Input: part model. Units: mm. Frame: model coordinates. Face numbers are marked on the shaded views. A direction names the side the tool comes from. Coordinates: 2 decimals unless noted, no trailing zeros. Order: outer loops, then holes, each group sorted by start corner. A loop starts at its lowest first (then second) coordinate and runs counter-clockwise, first axis right, second up. Notation, with made-up numbers: (68, 74.5) -> (98, 74.5) arc R26 cw to (98, 95.5) -> close; hole circle Ø7 at (-32, 37). An arc over 180 degrees is marked (long way). One line per question, with ' | ' between items.
```python
from build123d import *

# Parameters (mm, degrees)
SKETCH1_R           = 40
BOSS_EXTRUDE1_DEPTH = 3
SKETCH2_R           = 30
BOSS_EXTRUDE2_DEPTH = 18
SKETCH3_R           = 1.625
SKETCH3_R_2         = 11.5
SKETCH3_R_3         = 2.5
CUT_EXTRUDE1_DEPTH  = 61.340699366


with BuildPart() as part:
    # Sketch1 → Boss-Extrude1 (new body)
    with BuildSketch(Plane.XY):
        Circle(SKETCH1_R)
    extrude(amount=BOSS_EXTRUDE1_DEPTH)

    # Sketch2 → Boss-Extrude2 (add)
    with BuildSketch(Plane.XY.offset(3)):
        Circle(SKETCH2_R)
    extrude(amount=BOSS_EXTRUDE2_DEPTH)

    # Sketch3 → Cut-Extrude1 (cut, through all)
    with BuildSketch(Plane.XY.offset(21)):
        with Locations((0, 20)):
            Circle(SKETCH3_R)
        with Locations((17.320508076, -10)):
            Circle(SKETCH3_R)
        with Locations((-17.320508076, -10)):
            Circle(SKETCH3_R)
        Circle(SKETCH3_R_2)
        with Locations((0, -20)):
            Circle(SKETCH3_R_3)
    extrude(amount=-CUT_EXTRUDE1_DEPTH, mode=Mode.SUBTRACT)


solid = part.part
```
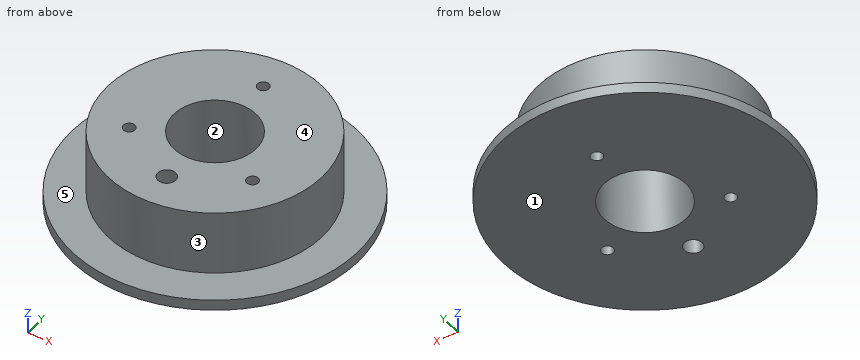
1. Pin query (flat end, axial travel): pin 1 Ø3 at (x, y) = (-17.32, -10) entering from +Z; pin 2 Ø4 at (y, z) = (6.5, 11.5) entering from -X; pin 3 Ø10 at (y, z) = (26.5, 9.5) entering from +X; pin 4 Ø4 at (x, z) = (-27, 15) entering from -Y. Return the tip coordinate at first contact, or that it passes through.
Recorded:
pin 1: passes through | pin 2: stops at x = -29.66 | pin 3: stops at x = 20.92 | pin 4: stops at y = -16.58
2. Mould query, pull axis X, two halves, no side actions, for the marked faces 1, 2 and 3. Classes: released by +X, released by -X, zero draft, split by the parting line, or undercut.
Recorded:
face 1: zero draft | face 2: undercut | face 3: split by the parting line
3. Access query for the marked faces 4 and 5. Directions: +Z, -Z, +X, -X, +Y, -Y. A direction counts if a zero-diameter tool reaches every point of the face in a straight line with its end or side. Return the directions, or none.
Recorded:
face 4: +Z, +X, -X, +Y, -Y | face 5: +Z
4. Cut plane A-A, the plane x = 0. Return loops of the section in (y, z) (3 decimals).
Recorded:
outline: (-40, 0) -> (-22.5, 0) -> (-22.5, 21) -> (-30, 21) -> (-30, 3) -> (-40, 3) -> close; (-17.5, 0) -> (-11.5, 0) -> (-11.5, 21) -> (-17.5, 21) -> close; (11.5, 0) -> (18.375, 0) -> (18.375, 21) -> (11.5, 21) -> close; (21.625, 0) -> (40, 0) -> (40, 3) -> (30, 3) -> (30, 21) -> (21.625, 21) -> close
5. Ray query, line 1 (Y direction, x = 0, z = 10) (3 decimals); line 2 (Y direction, x = -2, z = 6.25); line 3 (Y direction, x = -16, z = 15.5). Return the intervals inside material, ascending. Write a range as [from, to].
Recorded:
line 1: y = [-30, -22.5], [-17.5, -11.5], [11.5, 18.375], [21.625, 30] | line 2: y = [-29.93, -21.5], [-18.5, -11.32], [11.32, 29.93] | line 3: y = [-25.38, -10.95], [-9.05, 25.38]
6. Cut plane B-B, the plane z = 11.75. State how many separate pieces and enclosed holes the cut face has, and give its area (3 significant figures).
Recorded:
separate pieces: 1 | enclosed holes: 5 | area: 2,370 mm^2
7. Cut plane D-D, the plane y = 20. Return loops of the section in (x, z) (3 decimals).
Recorded:
outline: (-34.641, 0) -> (-1.625, 0) -> (-1.625, 21) -> (-22.361, 21) -> (-22.361, 3) -> (-34.641, 3) -> close; (1.625, 0) -> (34.641, 0) -> (34.641, 3) -> (22.361, 3) -> (22.361, 21) -> (1.625, 21) -> close
8. Cut plane C-C, the plane x = 9. Return loops of the section in (y, z).
Recorded:
outline: (-38.97, 0) -> (-7.16, 0) -> (-7.16, 21) -> (-28.62, 21) -> (-28.62, 3) -> (-38.97, 3) -> close; (7.16, 0) -> (38.97, 0) -> (38.97, 3) -> (28.62, 3) -> (28.62, 21) -> (7.16, 21) -> close
